Verification items for this drawing (mm, ordinates from the low corner). A direction names the side the tool comes from. Give positions to 0.01 mm unless a question says otherwise; leave off trailing zeros. Write each loop counter-clockwise with the first axis right and the second up, starting at its lowest first coordinate (ties: lowest second). Pieces come first, ordered by that corner, then holes. Notation, with made-up numbers: M -37.75,73.25 L 1.25,73.25 A31 cw 1.25,99.25 Z; hole C -35.5,48 d11. An arc over 180 degrees is marked long. Write each question's results on one line, items separated by ' | '.
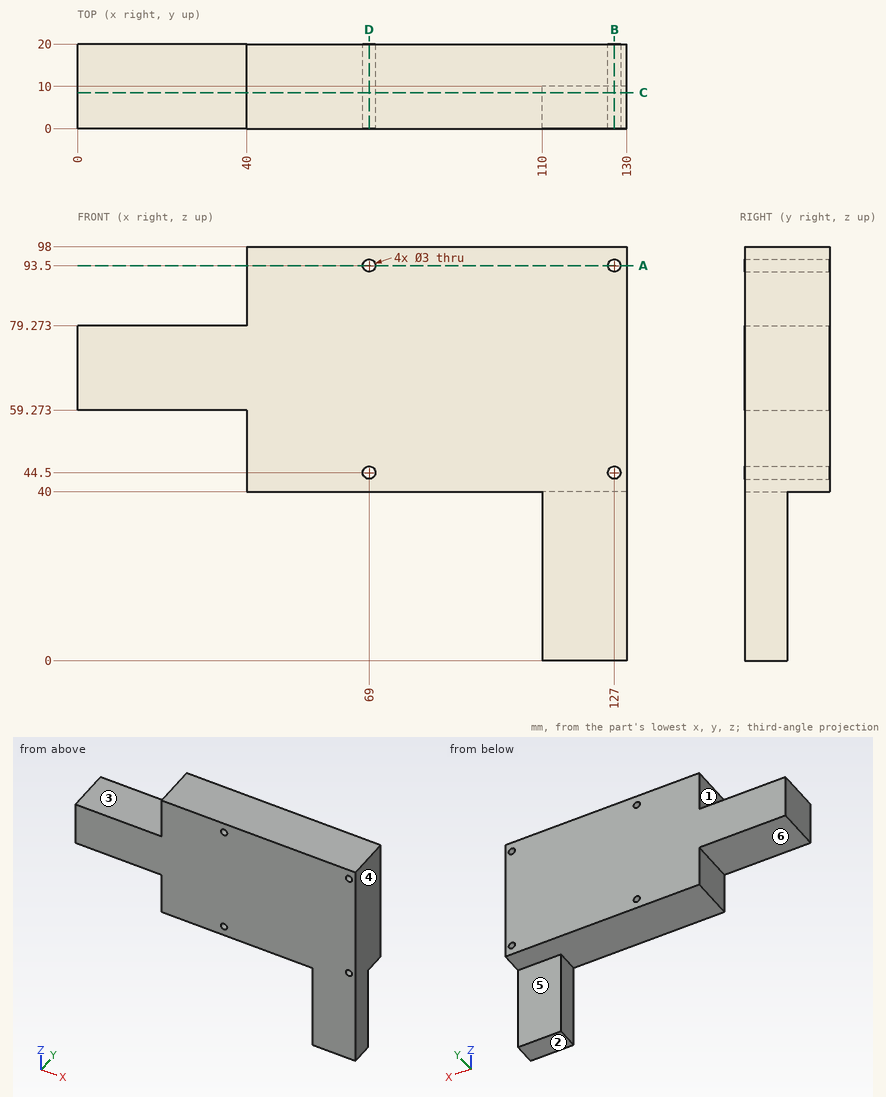
Q1. Section check A-A (z = 93.5). Enter the section's corners in (x, y), then the cut area to 3 significant figures.
Answer key:
outline: M 40,0 L 67.5,0 L 67.5,20 L 40,20 Z; M 70.5,0 L 125.5,0 L 125.5,20 L 70.5,20 Z; M 128.5,0 L 130,0 L 130,20 L 128.5,20 Z | area: 1,680 mm2
Q2. Release check for a two-part mould opening along Z. For the marked faces 1, 2 and 3 record: released by +Z, released by -Z, zero draft, split by the parting line, or undercut.
Answer key:
face 1: zero draft | face 2: released by -Z | face 3: released by +Z
Q3. Material ranges on probe 1 along X at (y, z) = (14.5, 93.5); probe 2 along Z at (x, y) = (69, 9); probe 3 along Z at (x, y) = (70, 3.25), recorded low to high. Write a range as [from, to].
Answer key:
probe 1: x = [40, 67.5], [70.5, 125.5], [128.5, 130] | probe 2: z = [40, 43], [46, 92], [95, 98] | probe 3: z = [40, 43.38], [45.62, 92.38], [94.62, 98]
Q4. Depth check by flat-ended pin: P1, Ø3, axis at x = 111, z = 37.5, coming from the +Y side; P2, Ø5.5, axis at y = 5.5, z = 87.5, coming from the -X side; P3, Ø1.8, axis at x = 69, z = 44.5, coming from the +Y side; P4, Ø10, axis at x = 20, y = 11, coming from the -Z side. Enter the tip coordinate at first touch or a pass-through.
Answer key:
P1: stops at y = 10 | P2: stops at x = 40 | P3: passes through | P4: stops at z = 59.27
Q5. Section check B-B (x = 127). Enter the section's corners in (y, z), then the cut area to 3 significant figures.
Answer key:
outline: M 0,0 L 10,0 L 10,40 L 20,40 L 20,43 L 0,43 Z; M 0,46 L 20,46 L 20,92 L 0,92 Z; M 0,95 L 20,95 L 20,98 L 0,98 Z | area: 1,440 mm2
Q6. Section check C-C (y = 8.5). Enter the section's corners in (x, z).
Answer key:
outline: M 0,59.27 L 40,59.27 L 40,40 L 110,40 L 110,0 L 130,0 L 130,98 L 40,98 L 40,79.27 L 0,79.27 Z; hole C 69,44.5 d3; hole C 69,93.5 d3; hole C 127,44.5 d3; hole C 127,93.5 d3
Q7. Section check D-D (x = 69). Enter the section's corners in (y, z).
Answer key:
outline: M 0,40 L 20,40 L 20,43 L 0,43 Z; M 0,46 L 20,46 L 20,92 L 0,92 Z; M 0,95 L 20,95 L 20,98 L 0,98 Z
Q8. Access from +Z, -Z, +X, -X, +Y, -Y to the whole of each face (thin tool, end or side, straight path). Record for the marked faces 4, 5 and 6.
Answer key:
face 4: +Z, -Z, +X, +Y, -Y | face 5: -Z, +X, -X, +Y | face 6: -Z, -X, +Y, -Y
